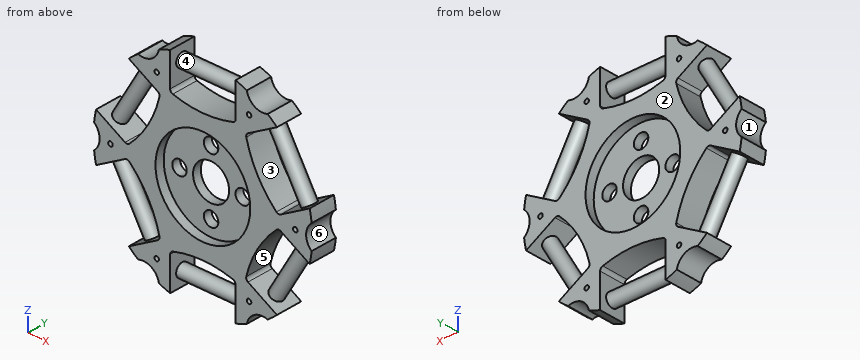
from build123d import *

# Parameters (mm, degrees)
SKETCH_1_W                  = 24.25
SKETCH_1_H                  = 5.9
CUT_EXTRUDE_1_DEPTH         = 35.798491347
CUT_EXTRUDE_2_DEPTH         = 35.798491347
CUT_EXTRUDE_3_DEPTH         = 35.798491347
CUT_EXTRUDE_4_DEPTH         = 35.798491347
CUT_EXTRUDE_5_DEPTH         = 35.798491347
CUT_EXTRUDE_6_DEPTH         = 35.798491347
CUT_EXTRUDE_7_DEPTH         = 35.798491347
CUT_EXTRUDE_8_DEPTH         = 35.034871823
CUT_EXTRUDE_9_DEPTH         = 35.034871823
CUT_EXTRUDE_10_DEPTH        = 35.034871823
CUT_EXTRUDE_11_DEPTH        = 34.930864282
CUT_EXTRUDE_12_DEPTH        = 34.930864282
SKETCH_15_W                 = 14.5
SKETCH_15_H                 = 1.5
HOLE_WIZARD_3_2_3_2_1_D     = 3.2
HOLE_WIZARD_3_2_3_2_1_DEPTH = 3.9
FILLET_1_R                  = 0.8
SKETCH_23_R                 = 0.5
CUT_EXTRUDE_13_DEPTH        = 10
PATTERN_CIRCULAR_1_COUNT    = 6
PATTERN_CIRCULAR_2_COUNT    = 6


with BuildPart() as part:
    # 草图1 → 旋转1 (revolve)
    with BuildSketch(Plane(origin=(0, 0, 0), x_dir=(-1, 0, 0), z_dir=(0, 0, -1)), mode=Mode.PRIVATE) as revolve_1_sk:
        with Locations((-12.125, -0.05)):
            Rectangle(SKETCH_1_W, SKETCH_1_H)
    revolve(revolve_1_sk.sketch.rotate(Axis((0, -3, 0), (0, 1, 0)), 270), axis=Axis((0, -3, 0), (0, 1, 0)))

    # 草图2 → 切除-拉伸1 (cut, through all)
    with BuildSketch(Plane(origin=(0, 2.9, 0), x_dir=(-1, 0, 0), z_dir=(0, 1, 0))):
        with BuildLine():
            Line((-7.25, 23.140872931), (-7.25, 15.140872931))
            ThreePointArc((-7.25, 15.140872931), (0, 14), (7.25, 15.140872931))
            Line((7.25, 15.140872931), (7.25, 23.140872931))
            ThreePointArc((7.25, 23.140872931), (0, 24.25), (-7.25, 23.140872931))
        make_face()
    extrude(amount=-CUT_EXTRUDE_1_DEPTH, mode=Mode.SUBTRACT)

    # 草图3 → 切除-拉伸2 (cut, through all)
    with BuildSketch(Plane(origin=(0, 2.9, 0), x_dir=(-1, 0, 0), z_dir=(0, 1, 0))):
        with BuildLine():
            ThreePointArc((14.354448547, 19.545135121), (12.125, 21.001116042), (9.749359262, 22.20388466))
            ThreePointArc((9.749359262, 22.20388466), (11.44, 19.814661239), (14.354448547, 19.545135121))
        make_face()
    extrude(amount=-CUT_EXTRUDE_2_DEPTH, mode=Mode.SUBTRACT)

    # 草图4 → 切除-拉伸3 (cut, through all)
    with BuildSketch(Plane(origin=(0, 2.9, 0), x_dir=(-1, 0, 0), z_dir=(0, 1, 0))):
        with BuildLine():
            Line((16.415583824, 17.849120643), (9.487380594, 13.849120643))
            ThreePointArc((9.487380594, 13.849120643), (12.124355653, 7), (16.737380594, 1.291752288))
            Line((16.737380594, 1.291752288), (23.665583824, 5.291752288))
            ThreePointArc((23.665583824, 5.291752288), (21.001116042, 12.125), (16.415583824, 17.849120643))
        make_face()
    extrude(amount=-CUT_EXTRUDE_3_DEPTH, mode=Mode.SUBTRACT)

    # 草图5 → 切除-拉伸4 (cut, through all)
    with BuildSketch(Plane(origin=(0, 2.9, 0), x_dir=(-1, 0, 0), z_dir=(0, 1, 0))):
        with BuildLine():
            ThreePointArc((24.103807809, -2.658749539), (24.25, 0), (24.103807809, 2.658749539))
            ThreePointArc((24.103807809, 2.658749539), (22.88, 0), (24.103807809, -2.658749539))
        make_face()
    extrude(amount=-CUT_EXTRUDE_4_DEPTH, mode=Mode.SUBTRACT)

    # 草图6 → 切除-拉伸5 (cut, through all)
    with BuildSketch(Plane(origin=(0, 2.9, 0), x_dir=(-1, 0, 0), z_dir=(0, 1, 0))):
        with BuildLine():
            Line((23.665583824, -5.291752288), (16.737380594, -1.291752288))
            ThreePointArc((16.737380594, -1.291752288), (12.124355653, -7), (9.487380594, -13.849120643))
            Line((9.487380594, -13.849120643), (16.415583824, -17.849120643))
            ThreePointArc((16.415583824, -17.849120643), (21.001116042, -12.125), (23.665583824, -5.291752288))
        make_face()
    extrude(amount=-CUT_EXTRUDE_5_DEPTH, mode=Mode.SUBTRACT)

    # 草图7 → 切除-拉伸6 (cut, through all)
    with BuildSketch(Plane(origin=(0, 2.9, 0), x_dir=(-1, 0, 0), z_dir=(0, 1, 0))):
        with BuildLine():
            ThreePointArc((9.749359262, -22.20388466), (12.125, -21.001116042), (14.354448547, -19.545135121))
            ThreePointArc((14.354448547, -19.545135121), (11.44, -19.814661239), (9.749359262, -22.20388466))
        make_face()
    extrude(amount=-CUT_EXTRUDE_6_DEPTH, mode=Mode.SUBTRACT)

    # 草图8 → 切除-拉伸7 (cut, through all)
    with BuildSketch(Plane(origin=(0, 2.9, 0), x_dir=(-1, 0, 0), z_dir=(0, 1, 0))):
        with BuildLine():
            Line((7.25, -23.140872931), (7.25, -15.140872931))
            ThreePointArc((7.25, -15.140872931), (0, -14), (-7.25, -15.140872931))
            Line((-7.25, -15.140872931), (-7.25, -23.140872931))
            ThreePointArc((-7.25, -23.140872931), (0, -24.25), (7.25, -23.140872931))
        make_face()
    extrude(amount=-CUT_EXTRUDE_7_DEPTH, mode=Mode.SUBTRACT)

    # 草图9 → 切除-拉伸8 (cut, through all)
    with BuildSketch(Plane(origin=(0, 2.9, 0), x_dir=(-1, 0, 0), z_dir=(0, 1, 0))):
        with BuildLine():
            ThreePointArc((-14.354448547, -19.545135121), (-12.125, -21.001116042), (-9.749359262, -22.20388466))
            ThreePointArc((-9.749359262, -22.20388466), (-11.44, -19.814661239), (-14.354448547, -19.545135121))
        make_face()
    extrude(amount=-CUT_EXTRUDE_8_DEPTH, mode=Mode.SUBTRACT)

    # 草图10 → 切除-拉伸9 (cut, through all)
    with BuildSketch(Plane(origin=(0, 2.9, 0), x_dir=(-1, 0, 0), z_dir=(0, 1, 0))):
        with BuildLine():
            Line((-16.415583824, -17.849120643), (-9.487380594, -13.849120643))
            ThreePointArc((-9.487380594, -13.849120643), (-12.124355653, -7), (-16.737380594, -1.291752288))
            Line((-16.737380594, -1.291752288), (-23.665583824, -5.291752288))
            ThreePointArc((-23.665583824, -5.291752288), (-21.001116042, -12.125), (-16.415583824, -17.849120643))
        make_face()
    extrude(amount=-CUT_EXTRUDE_9_DEPTH, mode=Mode.SUBTRACT)

    # 草图11 → 切除-拉伸10 (cut, through all)
    with BuildSketch(Plane(origin=(0, 2.9, 0), x_dir=(-1, 0, 0), z_dir=(0, 1, 0))):
        with BuildLine():
            ThreePointArc((-24.103807809, 2.658749539), (-24.25, 0), (-24.103807809, -2.658749539))
            ThreePointArc((-24.103807809, -2.658749539), (-22.88, 0), (-24.103807809, 2.658749539))
        make_face()
    extrude(amount=-CUT_EXTRUDE_10_DEPTH, mode=Mode.SUBTRACT)

    # 草图12 → 切除-拉伸11 (cut, through all)
    with BuildSketch(Plane(origin=(0, 2.9, 0), x_dir=(-1, 0, 0), z_dir=(0, 1, 0))):
        with BuildLine():
            Line((-23.665583824, 5.291752288), (-16.737380594, 1.291752288))
            ThreePointArc((-16.737380594, 1.291752288), (-12.124355653, 7), (-9.487380594, 13.849120643))
            Line((-9.487380594, 13.849120643), (-16.415583824, 17.849120643))
            ThreePointArc((-16.415583824, 17.849120643), (-21.001116042, 12.125), (-23.665583824, 5.291752288))
        make_face()
    extrude(amount=-CUT_EXTRUDE_11_DEPTH, mode=Mode.SUBTRACT)

    # 草图13 → 切除-拉伸12 (cut, through all)
    with BuildSketch(Plane(origin=(0, 2.9, 0), x_dir=(-1, 0, 0), z_dir=(0, 1, 0))):
        with BuildLine():
            ThreePointArc((-9.749359262, 22.20388466), (-12.125, 21.001116042), (-14.354448547, 19.545135121))
            ThreePointArc((-14.354448547, 19.545135121), (-11.44, 19.814661239), (-9.749359262, 22.20388466))
        make_face()
    extrude(amount=-CUT_EXTRUDE_12_DEPTH, mode=Mode.SUBTRACT)

    # 草图14 → 切除-旋转1 (revolve, cut)
    with BuildSketch(Plane.XY):
        Polygon((10.5, 2.9), (0, 2.9), (0, -3), (10.5, -3), (10.5, -1), (4, -1), (4, 0.9), (10.5, 0.9), align=None)
    revolve(axis=Axis((0, 2.9, 0), (0, -1, 0)), mode=Mode.SUBTRACT)

    # 草图15 → 旋转2 (revolve)
    with BuildSketch(Plane(origin=(0, 0, 20), x_dir=(-1, 0, 0), z_dir=(0, 0, -1)), mode=Mode.PRIVATE) as revolve_2_sk:
        with Locations((0, 0.7)):
            Rectangle(SKETCH_15_W, SKETCH_15_H)
    revolve_2 = revolve(revolve_2_sk.sketch.rotate(Axis((7.25, -0.05, 20), (-1, 0, 0)), 270), axis=Axis((7.25, -0.05, 20), (-1, 0, 0)))

    # Ø3.2 (3.2) 直径孔1
    with Locations(Plane(origin=(0, -1, 0), x_dir=(-1, 0, 0), z_dir=(0, -1, 0))):
        with Locations((0, 7), (0, -7), (-7, 0), (7, 0)):
            Hole(HOLE_WIZARD_3_2_3_2_1_D / 2, depth=HOLE_WIZARD_3_2_3_2_1_DEPTH)

    # 圆角1
    fillet_1_edges = [part.edges().sort_by_distance(p)[0] for p in [
        (16.737380594, -0.05, -1.291752288),
        (9.487380594, -0.05, -13.849120643),
        (-7.25, -0.05, 15.140872931),
        (7.25, -0.05, 15.140872931),
        (9.487380594, -0.05, 13.849120643),
        (16.737380594, -0.05, 1.291752288),
        (-16.737380594, -0.05, 1.291752288),
        (-9.487380594, -0.05, 13.849120643),
        (-9.487380594, -0.05, -13.849120643),
        (-16.737380594, -0.05, -1.291752288),
        (7.25, -0.05, -15.140872931),
        (-7.25, -0.05, -15.140872931),
    ]]
    fillet(fillet_1_edges, radius=FILLET_1_R)

    # 草图23 → 切除-拉伸13 (cut)
    with BuildSketch(Plane.XZ.offset(3)):
        with Locations(Location((20.48, 0, 0), (0, 0, 270))):
            Circle(SKETCH_23_R)
    cut_extrude_13 = extrude(amount=-CUT_EXTRUDE_13_DEPTH, mode=Mode.SUBTRACT)

    # 阵列(圆周)1: 切除-拉伸13 ×6 about axis
    pattern_circular_1_axis = Axis((0, 0, 0), (0, 1, 0))
    for i in range(1, PATTERN_CIRCULAR_1_COUNT):
        add(cut_extrude_13.rotate(pattern_circular_1_axis, i * 360 / PATTERN_CIRCULAR_1_COUNT), mode=Mode.SUBTRACT)

    # 阵列(圆周)2: 旋转2 ×6 about axis
    pattern_circular_2_axis = Axis((0, 2.9, 0), (0, -1, 0))
    for i in range(1, PATTERN_CIRCULAR_2_COUNT):
        add(revolve_2.rotate(pattern_circular_2_axis, i * 360 / PATTERN_CIRCULAR_2_COUNT))


solid = part.part
Input: part model. Units: mm. Frame: model coordinates. Face numbers are marked on the shaded views. A direction names the side the tool comes from. Give positions to 0.01 mm unless a question says otherwise; leave off trailing zeros. Order: outer loops, then holes, each group sorted by start corner. A loop starts at its lowest first (then second) coordinate and runs counter-clockwise, first axis right, second up.
Q1. Set-up query: the marked faces 4, 5 and 6. Return all of +Z, -Z, +X, -X, +Y, -Y with unobstructed straight access to the full face (end or side cutting, diameter ignored); none if empty.
Checked values:
face 4: none
face 5: +Y, -Y
face 6: +X, +Y, -Y
Q2. Draft query along X for the marked faces 1, 2 and 3. Return one class per face: +X half, -X half, draft (parallel to the pull), parting line (faces both ways), or undercut.
Checked values:
face 1: -X half
face 2: draft
face 3: undercut
Q3. Ray query, probe 1 along X at (y, z) = (-0.15, -18); probe 2 along X at (y, z) = (0.4, 6); probe 3 along Z at (x, y) = (7, 1.2). Return the intervals inside material, ascending.
Checked values:
probe 1: x = -16.25 to -10.66, -9.82 to -7.25, 7.25 to 9.82, 10.66 to 16.25
probe 2: x = -21.28 to -17.98, -12.74 to -1.25, 1.25 to 12.74, 17.98 to 21.28
probe 3: z = -20.83 to -19.17, -15.15 to -7.83, 7.83 to 15.15, 19.17 to 20.83
Q4. Section C-C on z = 7. State how many separate pieces and enclosed holes the cut face has, and give its area (3 significant figures).
Checked values:
separate pieces: 4
enclosed holes: 0
area: 90.7 mm2
Q5. Section B-B on x = 6. Output: boundary loops of the cut face in (y, z), and give its area (3 significant figures).
Checked values:
outline: (-3, -14.78) - (2.9, -14.78) - (2.9, -8.62) - (0.9, -8.62) - (0.9, -1.25) - (-1, -1.25) - (-1, -8.62) - (-3, -8.62) - close; (-3, 8.62) - (-1, 8.62) - (-1, 1.25) - (0.9, 1.25) - (0.9, 8.62) - (2.9, 8.62) - (2.9, 14.78) - (-3, 14.78) - close; circle Ø3 at (-0.05, -20); circle Ø3 at (-0.05, 20)
area: 115 mm2
Q6. Contact query for flat-ended pins moving along their axis: pin 1 Ø1 at (x, y) = (4.5, -2.5) entering from -Z; pin 2 Ø10.5 at (x, z) = (-1, -1) entering from +Y; pin 3 Ø1.8 at (y, z) = (1, -21) entering from -X. Output: stop coordinate, or through.
Checked values:
pin 1: stops at z = -14.54
pin 2: stops at y = 0.9
pin 3: stops at x = -11.02
Q7. Section A-A on x = 0. Output: boundary loops of the cut face in (y, z), and give its area (3 significant figures).
Checked values:
outline: (-3, -14) - (2.9, -14) - (2.9, -10.5) - (0.9, -10.5) - (0.9, -8.6) - (-1, -8.6) - (-1, -10.5) - (-3, -10.5) - close; (-3, 10.5) - (-1, 10.5) - (-1, 8.6) - (0.9, 8.6) - (0.9, 10.5) - (2.9, 10.5) - (2.9, 14) - (-3, 14) - close; circle Ø3 at (-0.05, -20); circle Ø3 at (-0.05, 20); (-1, -5.4) - (0.9, -5.4) - (0.9, -4) - (-1, -4) - close; (-1, 4) - (0.9, 4) - (0.9, 5.4) - (-1, 5.4) - close
area: 68.0 mm2
